Part print with two shaded views. Sizes in mm from the minimum x, y, z corner. Round coordinates to 2 decimals unless told otherwise and drop trailing zeros. Loops run counter-clockwise (first coordinate to the right, second up) from the corner with the lowest first, then second, coordinate; pieces in that order, holes last. Notation, with made-up numbers: M 15.25,17.5 L 58.25,17.5 A19 ccw 58.25,24.5 Z; hole C 49.25,-2.5 d4. An arc over 180 degrees is marked long. Use a Markdown table: item, result. Add a question column.
Item 1: Saw through at A-A on y = 201. Write the cut outline in (x, z), then the cut area to 3 significant figures.
Item 2: Wall check: L1, parallel to X at y = 216.5, z = 2; L2, parallel to X at y = 271, z = 11; L3, parallel to Y at x = 425, z = 7.5. Give the ranges that are in metal, low to high. Write a range as from..to.
Item 3: Saw through at C-C on y = 279.5. Write the cut outline in (x, z).
Item 4: Saw through at B-B on z = 6.5. Write the cut outline in (x, y).
Item 5: Saw through at D-D on x = 397. Write the cut outline in (y, z), then the cut area to 3 significant figures.
Item 6: Pin check, flat tips, straight feed: P1, Ø4, axis at x = 38.5, z = 6, coming from the -Y side; P2, Ø1.5, axis at x = 256, z = 10.5, coming from the -Y side. Stop position of each tip, or through.
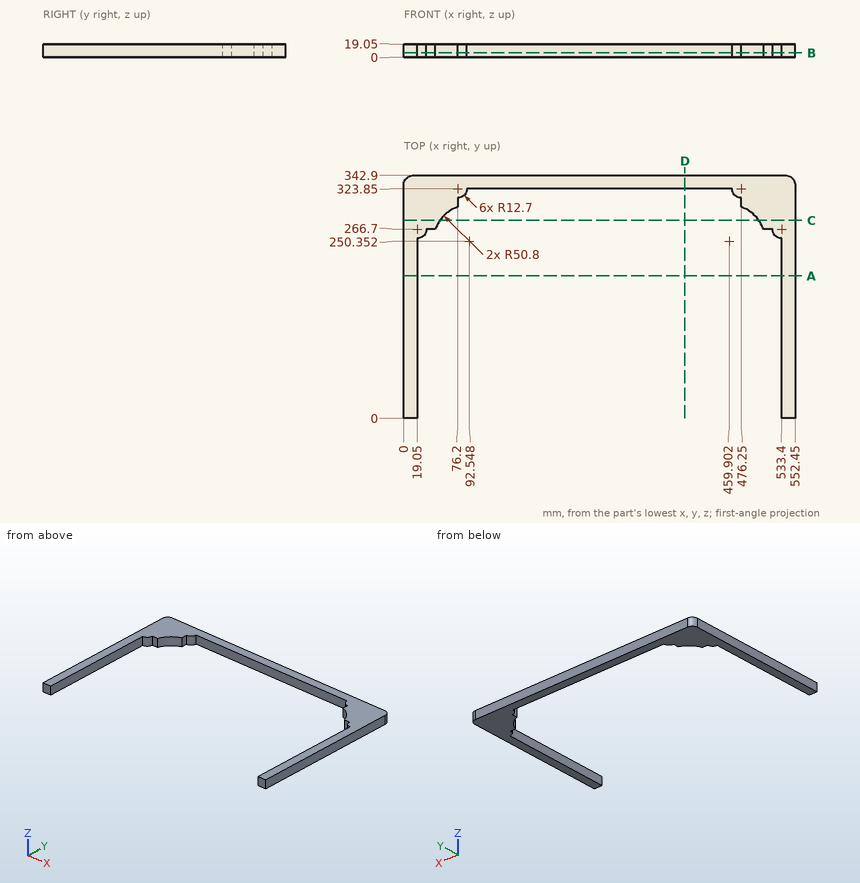
Entries:
| question | item | result |
|---|---|---|
| 1 | outline | M 0,0 L 19.05,0 L 19.05,19.05 L 0,19.05 Z; M 533.4,0 L 552.45,0 L 552.45,19.05 L 533.4,19.05 Z |
| 1 | area | 726 mm2 |
| 2 | L1 | 0..19.05, 533.4..552.45 |
| 2 | L2 | 0..46.13, 506.32..552.45 |
| 2 | L3 | 323.85..342.9 |
| 3 | outline | M 0,0 L 50.94,0 L 50.94,19.05 L 0,19.05 Z; M 501.51,0 L 552.45,0 L 552.45,19.05 L 501.51,19.05 Z |
| 4 | outline | M 0,0 L 19.05,0 L 19.05,254 A12.7 ccw 31.75,266.7 L 44.45,266.7 A50.8 cw 76.2,298.45 L 76.2,311.15 A12.7 ccw 88.9,323.85 L 463.55,323.85 A12.7 ccw 476.25,311.15 L 476.25,298.45 A50.8 cw 508,266.7 L 520.7,266.7 A12.7 ccw 533.4,254 L 533.4,0 L 552.45,0 L 552.45,330.2 A12.7 ccw 539.75,342.9 L 12.7,342.9 A12.7 ccw 0,330.2 Z |
| 5 | outline | M 323.85,0 L 342.9,0 L 342.9,19.05 L 323.85,19.05 Z |
| 5 | area | 363 mm2 |
| 6 | P1 | y = 266.7 |
| 6 | P2 | y = 323.85 |
